Input: dimensioned drawing with shaded views. Units: mm. Origin: part minimum x, y, z. A direction names the side the tool comes from. Give positions to 0.01 mm unless a question says otherwise; leave off trailing zeros. Write each loop counter-clockwise with the first axis right and the second up, starting at its lowest first coordinate (ties: lowest second). Pieces come first, ordered by that corner, then holes. Notation, with made-up numbers: M 49.25,48 L 62.25,48 A24 cw 62.25,71 Z; hole C 63.5,25 d10. An arc over 180 degrees is marked long. Answer as a JSON object with one key per item and string values.
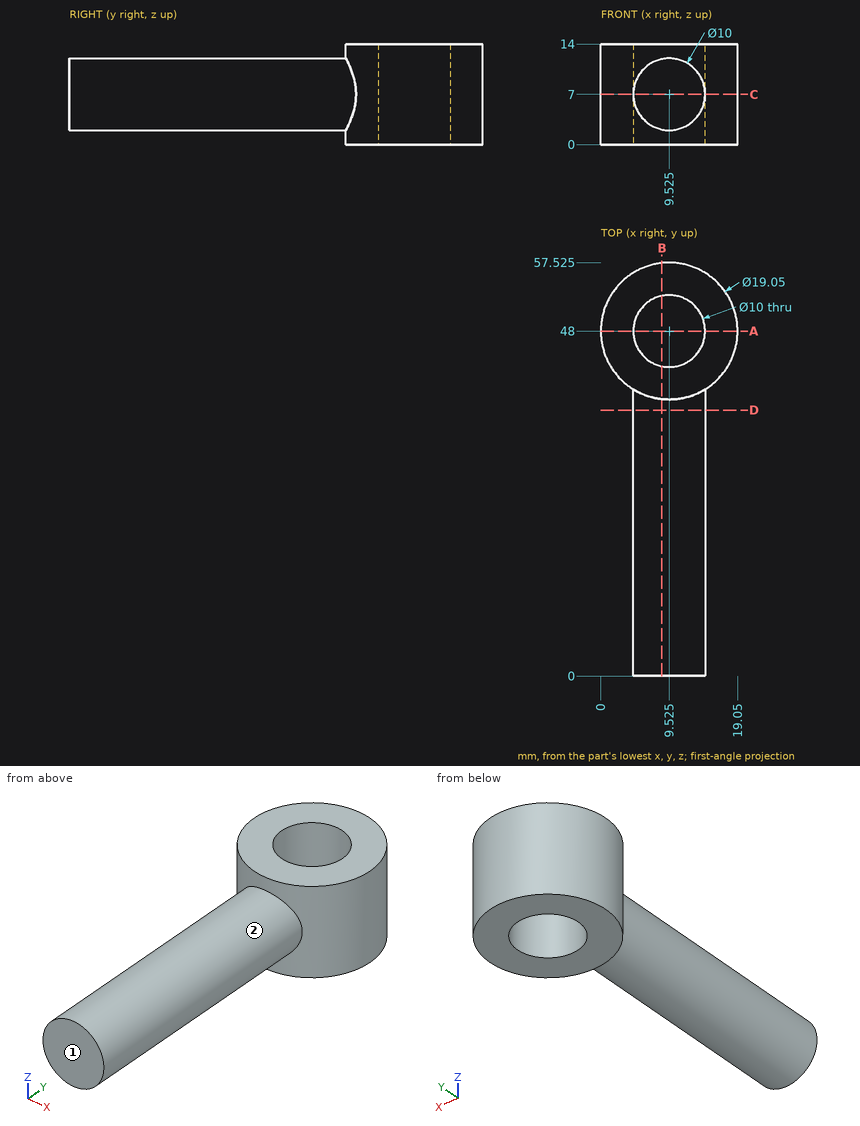
1) Set-up query: the marked faces 1 and 2. Return all of +Z, -Z, +X, -X, +Y, -Y with unobstructed straight access to the full face (end or side cutting, diameter ignored); none if empty.
Geometry check:
{"face 1": "+Z, -Z, +X, -X, -Y", "face 2": "-Y"}
2) Cut plane A-A on y = 48. Return loops of the section in (x, z) (3 decimals).
Geometry check:
{"outline": "M 0,0 L 4.525,0 L 4.525,14 L 0,14 Z; M 14.525,0 L 19.05,0 L 19.05,14 L 14.525,14 Z"}
3) Cut plane C-C on z = 7. Return loops of the section in (x, y) (3 decimals), and give its area (3 significant figures).
Geometry check:
{"outline": "M 4.525,0 L 14.525,0 L 14.525,39.893 A9.525 ccw long 4.525,39.893 Z; hole C 9.525,48 d10", "area": "596 mm2"}
4) Cut plane B-B on x = 8.5. Return loops of the section in (y, z), and give its area (3 significant figures).
Geometry check:
{"outline": "M 0,2.11 L 38.53,2.11 L 38.53,0 L 43.11,0 L 43.11,14 L 38.53,14 L 38.53,11.89 L 0,11.89 Z; M 52.89,0 L 57.47,0 L 57.47,14 L 52.89,14 Z", "area": "505 mm2"}
5) Contact query for flat-ended pins moving along their axis: P1, Ø6, axis at y = 6.5, z = 3, coming from the +X side; P2, Ø2, axis at y = 44.5, z = 1.5, coming from the +X side; P3, Ø1, axis at x = 10.5, y = 33.5, coming from the -Z side. Output: stop coordinate, or through.
Geometry check:
{"P1": "stops at x = 14.42", "P2": "stops at x = 18.72", "P3": "stops at z = 2.02"}
6) Line query: line 1 (Y direction, x = 9.25, z = 10.5); line 2 (Y direction, x = 7.25, z = 4); line 3 (Z direction, x = 13.25, y = 30). Output: solid intervals per line, ascending. Write a range as from..to.
Geometry check:
{"line 1": "y = 0..43.01, 52.99..57.52", "line 2": "y = 0..43.55, 52.45..57.25", "line 3": "z = 3.66..10.34"}
7) Cut plane D-D on y = 37. Return loops of the section in (x, z) (3 decimals), and give its area (3 significant figures).
Geometry check:
{"outline": "C 9.525,7 d10", "area": "78.5 mm2"}
